CAD build for the part. Positions are in the model's coordinates, mm. Face numbers are marked on the shaded views. A direction names the side the tool comes from. Coordinates: 2 decimals unless noted, no trailing zeros. Loops run counter-clockwise (first coordinate to the right, second up) from the corner with the lowest first, then second, coordinate; pieces in that order, holes last. Notation, with made-up numbers: (68.25, -19) - (75.25, -19) arc R24 ccw to (75.25, -5) - close; hole circle Ø6 at (-11.5, 77). An arc over 180 degrees is marked (long way). Put each result on its own line as item: value.
Autodesk Inventor part; units mm, degrees
ref_plane "YZ Plane" through (0, 0, 0) normal (1, 0, 0) x (0, 1, 0)
ref_plane "XZ Plane" through (0, 0, 0) normal (0, 1, 0) x (-1, 0, 0)
ref_plane "XY Plane" through (0, 0, 0) normal (0, 0, 1) x (1, 0, 0)
sketch "Sketch1" plane through (0, 0, 0) normal (0, 1, 0) x (-1, 0, 0)
  circle A0 centre (0, 0) radius 135
  circle A1 centre (0, 0) radius 110
  circle A2 centre (0, 0) radius 125
  circle A3 centre (-125, 0) radius 3
  circle A4 centre (-101.1271, -73.4732) radius 3
  circle A5 centre (-38.6271, -118.8821) radius 3
  circle A6 centre (38.6271, -118.8821) radius 3
  circle A7 centre (101.1271, -73.4732) radius 3
  circle A8 centre (125, 0) radius 3
  circle A9 centre (101.1271, 73.4732) radius 3
  circle A10 centre (38.6271, 118.8821) radius 3
  circle A11 centre (-38.6271, 118.8821) radius 3
  circle A12 centre (-101.1271, 73.4732) radius 3
  dimension "d69" = 250
  dimension "d0" = 270
  dimension "d1" = 220
  dimension "d75" = 6
  dimension "d78" = 360
extrude "Extrusion1" add sketch "Sketch1" along normal mid plane 20 contours A0 | A8 A2 A7 A6 A5 A4 A3 A12 A11 A10 A9
sketch "Sketch4" plane through (0, 10, 0) normal (0, 1, 0) x (1, 0, 0)
  circle A0 centre (0, 0) radius 50.125
  circle A1 centre (0, 0) radius 135
  circle A2 centre (0, 0) radius 110
  line L0 (125.3494, 50.125) -> (150.3494, 50.125)
  line L1 (150.3494, 50.125) -> (150.3494, 35.125)
  line L2 (150.3494, 35.125) -> (125.3494, 35.125)
  line L3 (125.3494, 35.125) -> (125.3494, 50.125)
  line L4 (150.3494, 70.125) -> (104.7795, 70.125)
  line L5 (104.7795, 70.125) -> (104.7795, 85.125)
  line L6 (104.7795, 85.125) -> (150.3494, 85.125)
  line L7 (150.3494, 85.125) -> (150.3494, 70.125)
  line L8 (103.1497, 60.125) -> (138.3886, 60.125) construction
  point P0 (130.3504, 35.125)
  point P1 (115.3581, 70.125)
  dimension "d21" = 100.25
  dimension "d22" = 25
  dimension "d23" = 15
  dimension "d24" = 20
  dimension "d25" = 15
  dimension "d57" = 10
extrude "Extrusion3" add sketch "Sketch4" against normal up to surface (20 mm away) contours L6 L7 L4 A1 | A1 L0 L1 L2
fillet "Fillet1" radius 6 4 edges at (150.3494, 10, -77.625) (150.3494, -10, -77.625) (150.3494, -10, -42.625) (150.3494, 10, -42.625)
fillet "Fillet2" radius 10 1 edges at (104.7795, 0, -85.125)
fillet "Fillet3" radius 2 1 edges at (130.3504, 0, -35.125)
sketch "Sketch5" plane through (150.3494, -4, -85.125) normal (0, 0, -1) x (-1, 0, 0)
  line L0 (0, 8) -> (0, 0)
  line L1 (40.9135, -6) -> (6, -6)
  point P0 (150.3494, 4)
  point P1 (8, 4)
  point P2 (0, 4)
  dimension "d38" = 8
  dimension "d39" = 10
hole "Hole2" at (142.3494, 0, -85.125) direction (0, 0, 1) diameter 6 depth 50 counterbore diameter 9 counterbore depth 5
mirror "Mirror1" about plane through (0, 0, 0) normal (1, 0, 0) of "Extrusion3", "Fillet1", "Fillet2", "Fillet3", "Hole2"
mirror "Mirror2" about plane through (0, 0, 0) normal (0, 0, 1) of "Extrusion3", "Fillet1", "Fillet2", "Fillet3", "Hole2"
sketch "Sketch7" plane through (0, 10, 0) normal (0, 1, 0) x (1, 0, 0)
  line L0 (0, 0) -> (0, -158.0698) construction
  point P0 (0, -127.5)
  dimension "d50" = 127.5
hole "Hole3" at (0, 10, 127.5) direction (0, -1, 0) diameter 5 end through all
sketch "Sketch11" plane through (0, 10, 0) normal (0, 1, 0) x (1, 0, 0)
  line L0 (-158.7443, 70.125) -> (165.1324, 70.125)
  line L1 (165.1324, 70.125) -> (165.1324, -140.5382)
  line L2 (165.1324, -140.5382) -> (-158.7443, -140.5382)
  line L3 (-158.7443, -140.5382) -> (-158.7443, 70.125)
  point P0 (0, 0)
extrude "Extrusion7" cut sketch "Sketch11" against normal through all
fillet "Fillet7" radius 2 2 edges at (-84.7495, 0, -70.125) (84.7495, 0, -70.125)
properties part number "Cylinder 80-20 Spacer_2"
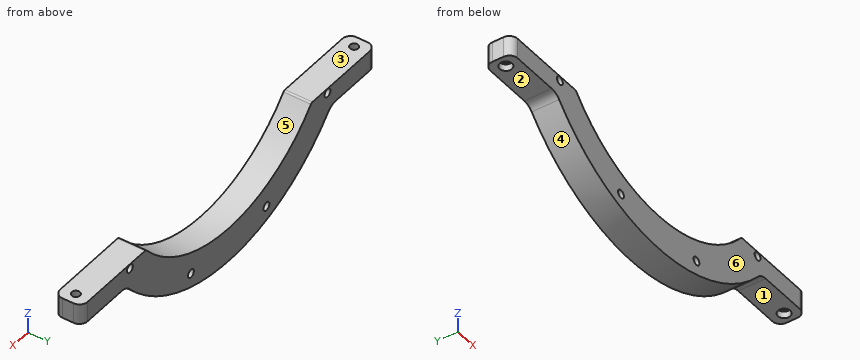
Q1. Slice it at C-C, the plane x = -47. Give the cut face in (y, z).
Determined:
outline: (-10, -126.55) - (10, -126.55) - (10, -99.45) - (-10, -99.45) - close
Q2. Pin check, flat tips, straight feed: pin 1 Ø7 at (x, y) = (-142.5, 1.5) entering from -Z (3 decimals); pin 2 Ø2 at (x, y) = (52, -4) entering from -Z; pin 3 Ø2 at (y, z) = (6, -86) entering from -X. Stop position of each tip, or through.
Determined:
pin 1: z = -85.125
pin 2: z = -125
pin 3: x = -150.15
Q3. Wall check: L1, parallel to X at y = 0, z = -74.75; L2, parallel to X at y = 7, z = -118; L3, parallel to Z at x = 132, y = 1.75 (3 decimals). Give the ranges that are in metal, low to high. Write a range as from..to.
Determined:
L1: -150.35..-145.35, -139.35..-103.84, -98.41..-80.7, 80.7..98.41, 103.84..139.35, 145.35..150.35
L2: -65.58..-41.49, -35.76..35.76, 41.49..65.58
L3: -85.125..-70.125
Q4. Slice it at B-B, the plane x = 130.5. Give the cut face in (y, z) (3 decimals), then the cut area to 3 significant figures.
Determined:
outline: (-10, -85.125) - (10, -85.125) - (10, -70.125) - (-10, -70.125) - close
area: 300 mm2
Q5. Tool access for the marked faces 1, 2 and 3: list every direction of +Z, -Z, +X, -X, +Y, -Y with a clear straight run to the whole face (end or side of a thin tool).
Determined:
face 1: -Z, +X, +Y, -Y
face 2: -Z, -X, +Y, -Y
face 3: +Z, +X, -X, +Y, -Y
Q6. Mould opens along X. For the marked faces 4, 5 and 6 say: +X half, -X half, draft (parallel to the pull), parting line (faces both ways), or undercut.
Determined:
face 4: parting line
face 5: undercut
face 6: draft
Q7. Slice it at A-A, the plane y = 0. State how many separate pieces and enclosed holes the cut face has, then the cut area to 3 significant figures.
Determined:
separate pieces: 3
enclosed holes: 4
area: 6,770 mm2
